```python
from build123d import *

# Parameters (mm, degrees)
EXTRUDE_1_DEPTH      = 2.5
EXTRUDE_1_DEPTH_BACK = 2.5
SKETCH_1_R           = 20


with BuildPart() as part:
    # Эскиз1 → Бобышка-Вытянуть1 (new, two sides: drawn at the far end of the back side and taken through both)
    with BuildSketch(Plane.XY.offset(-EXTRUDE_1_DEPTH_BACK)):
        with BuildLine():
            Line((-65, 5), (-27.279788924, 51.927451203))
            ThreePointArc((-27.279788924, 51.927451203), (0, 65), (27.279788924, 51.927451203))
            Line((27.279788924, 51.927451203), (65, 5))
            Line((65, 5), (65, 0))
            Line((65, 0), (-65, 0))
            Line((-65, 0), (-65, 5))
        make_face()
        with Locations((0, 30)):
            Circle(SKETCH_1_R, mode=Mode.SUBTRACT)
    extrude(amount=EXTRUDE_1_DEPTH + EXTRUDE_1_DEPTH_BACK)


solid = part.part
```
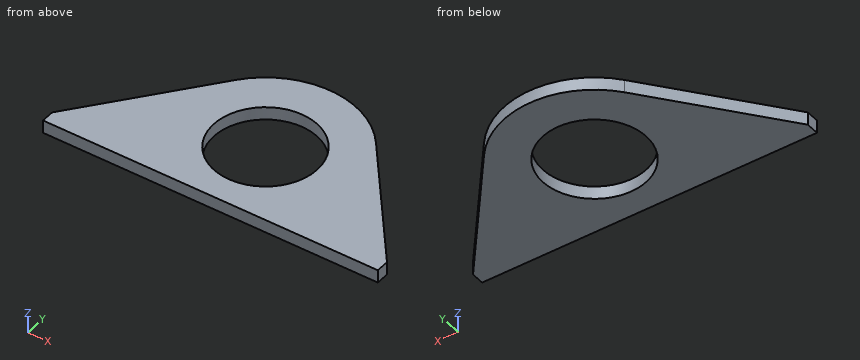
Can you work these out from the model? Positions are in its coordinate system, mm. Coordinates: 2 decimals unless noted, no trailing zeros. Loops run counter-clockwise (first coordinate to the right, second up) from the corner with the lowest first, then second, coordinate; pieces in that order, holes last. Notation, with made-up numbers: (-10.75, 7) - (41.25, 7) arc R13 cw to (41.25, 14) - close; hole circle Ø8 at (55, -16.75). An arc over 180 degrees is marked (long way). Answer as CSV lines item,"result". Start each with the question number.
1) Suppose I cut it at D-D (y = 58). Please give me the cut outline in (x, z), plus the area to 3 significant figures.
2) For pin 1 (2 mm diameter, centred on x = -50, y = 27.5, fed in from -Z), with a flat end and sliding along its axis, tell me the tip position at first contact or that it passes through.
3) Suppose I cut it at B-B (x = 10). Please give me the cut outline in (y, z), plus the area to 4 significant figures.
4) Suppose I cut it at C-C (y = 26). Please give me the cut outline in (x, z).
5) I need wall thicknesses on line 1 (Y direction, x = 0, z = 0.2); line 2 (Y direction, x = 5.5, z = -1.75); line 3 (X direction, y = 43, z = -2.05). Which ranges of each line are inside material? Lowest first, please. Write a range as from..to.
6) Suppose I cut it at A-A (z = -0.6). Please give me the cut outline in (x, y), plus the area to 3 significant figures.
Check result:
1,outline,"(-21, -2.5) - (21, -2.5) - (21, 2.5) - (-21, 2.5) - close"
1,area,"210 mm²"
2,pin 1,"passes through"
3,outline,"(0, -2.5) - (12.68, -2.5) - (12.68, 2.5) - (0, 2.5) - close; (47.32, -2.5) - (63.54, -2.5) - (63.54, 2.5) - (47.32, 2.5) - close"
3,area,"144.5 mm²"
4,outline,"(-48.12, -2.5) - (-19.6, -2.5) - (-19.6, 2.5) - (-48.12, 2.5) - close; (19.6, -2.5) - (48.12, -2.5) - (48.12, 2.5) - (19.6, 2.5) - close"
5,line 1,"y = 0..10, 50..65"
5,line 2,"y = 0..10.77, 49.23..64.57"
5,line 3,"x = -34.46..-15.2, 15.2..34.46"
6,outline,"(-65, 0) - (65, 0) - (65, 5) - (27.28, 51.93) arc R35 ccw to (-27.28, 51.93) - (-65, 5) - close; hole circle Ø40 at (0, 30)"
6,area,"4,220 mm²"
